Here's the drawing with two shaded views (mm, measured from the low corner). I have some questions. A direction names the side the tool comes from. Give positions to 0.01 mm unless a question says otherwise; leave off trailing zeros. Loops run counter-clockwise (first coordinate to the right, second up) from the corner with the lowest first, then second, coordinate; pieces in that order, holes last. Notation, with made-up numbers: M 11,10.25 L 51,10.25 A19 ccw 51,42.25 Z; hole C -30,-27.5 d2. An arc over 180 degrees is marked long. Put each result on its own line as item: value. Start each with the question number.
1) Imagine slicing it at C-C (x = 15). Write out the boundary of the cut face in (y, z) (1 decimal), then the cut area to 3 significant figures.
2) For the marked faces 4 and 5, which set-ups out of +Z, -Z, +X, -X, +Y, -Y let a thin tool reach every point of the face, with its end or its side?
3) Imagine slicing it at D-D (x = 21). Write out the boundary of the cut face in (y, z).
4) For P1, Ø0.8, axis at y = 3, z = 16, coming from the +X side; P2, Ø3, axis at x = 4.5, z = 8, coming from the -Y side; P3, Ø3, axis at x = 18.5, z = 17.5, coming from the +Y side; P4, Ø1.5, axis at x = 22, y = 1, coming from the +Z side, each with a flat end and sliding along its axis, tell me the tip position at first contact or that it passes through.
5) If we mould it in two halves opening along Z, with no side actions, what happens to the marked faces 1, 2 and 3? For each: +Z half, -Z half, draft (parallel to the pull), parting line (faces both ways), or undercut.
6) Imagine slicing it at B-B (z = 16.5). Write out the boundary of the cut face in (x, y).
7) Please list where these lines run through material, in increasing order: line 1 along X through (y, z) = (3.1, 20); line 2 along Z through (x, y) = (13, 2.85) (1 decimal); line 3 along Z through (x, y) = (16.5, 0.75). Write a range as from..to.
8) Imagine slicing it at A-A (y = 1.8). Write out the boundary of the cut face in (x, z) (1 decimal), then the cut area to 3 significant figures.
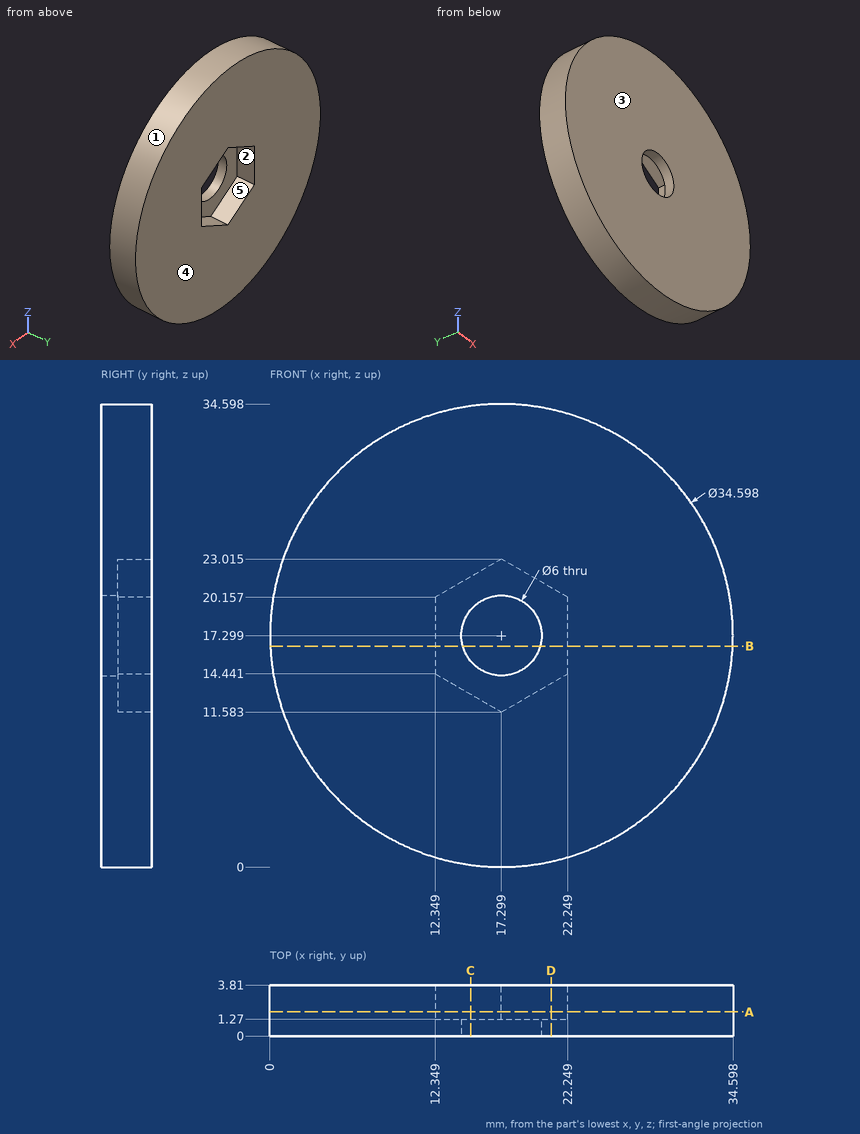
Recorded:
1. outline: M 0,0.2 L 3.8,0.2 L 3.8,12.9 L 1.3,12.9 L 1.3,15.4 L 0,15.4 Z; M 0,19.2 L 1.3,19.2 L 1.3,21.7 L 3.8,21.7 L 3.8,34.4 L 0,34.4 Z
1. area: 103 mm²
2. face 4: +Z, -Z, +X, -X, +Y
2. face 5: +Y
3. outline: M 0,0.4 L 3.81,0.4 L 3.81,13.72 L 1.27,13.72 L 1.27,20.88 L 3.81,20.88 L 3.81,34.2 L 0,34.2 Z
4. P1: x = 34.57
4. P2: y = 0
4. P3: through
4. P4: z = 34.14
5. face 1: parting line
5. face 2: undercut
5. face 3: draft
6. outline: M 0.02,0 L 14.41,0 L 14.41,1.27 L 12.35,1.27 L 12.35,3.81 L 0.02,3.81 Z; M 20.19,0 L 34.58,0 L 34.58,3.81 L 22.25,3.81 L 22.25,1.27 L 20.19,1.27 Z
7. line 1: 0.21..12.35, 22.25..34.39
7. line 2: 0.5..14.1, 20.5..34.1
7. line 3: 0.02..14.41, 20.19..34.58
8. outline: C 17.3,17.3 d34.6; hole M 12.3,14.4 L 17.3,11.6 L 22.2,14.4 L 22.2,20.2 L 17.3,23 L 12.3,20.2 Z
8. area: 855 mm²
